Could you check a few things on this model? Use its own coordinates, in mm. A direction names the side the tool comes from. Give positions to 0.01 mm unless a question says otherwise; leave off trailing zeros. Write each question's results on one line, items separated by ' | '. Start each with the question number.
1) On a 3-axis mill with a long thin cutter (end or side, diameter ignored), from which of +Z, -Z, +X, -X, +Y, -Y can I reach the whole of each face in a straight line? I mean faces 4 (the face through (-7, 20, -320)), 5 (the face through (-7, 0, 419)). Say none if no direction works.
2) If we mould it in two halves opening along Z, with no side actions, what happens to faces 1 (the face through (-7, 20, 320)), 2 (the face through (500, 74, 7)), 3 (the face through (-7, 74, -500))? For each: +Z half, -Z half, draft (parallel to the pull), parting line (faces both ways), or undercut.
3) I'm going to push a flat-ended pin straight in: pin 1 (20 mm diameter, centred on x = 121.5, z = 324, fed in from -Y). Where does the tip first touch, or does it pass through?
4) If I drill on probe 1 along Z at (x, y) = (-83, 13); probe 2 along Y at (x, z) = (-176, 331), over which ranges is the centre line in solid material (lowest first)? Write a range as [from, to].
from build123d import *

# Parameters (mm, degrees)
ESBO_O1_W                = 1000
ESBO_O1_H                = 1000
RESSALTO_EXTRUS_O1_DEPTH = 150
ESBO_O2_W                = 40
ESBO_O2_H                = 40
CORTE_EXTRUS_O1_DEPTH    = 1001


with BuildPart() as part:
    # Esboço1 → Ressalto-extrusão1 (new body)
    with BuildSketch(Plane(origin=(0, 0, 0), x_dir=(1, 0, 0), z_dir=(0, 1, 0))):
        Rectangle(ESBO_O1_W, ESBO_O1_H)
    extrude(amount=RESSALTO_EXTRUS_O1_DEPTH)

    # Esboço2 → Corte-extrusão1 (cut, through all)
    with BuildSketch(Plane.ZY.offset(500)):
        with Locations((320, 0)):
            Rectangle(ESBO_O2_W, ESBO_O2_H)
        with Locations((-320, 0)):
            Rectangle(ESBO_O2_W, ESBO_O2_H)
    extrude(amount=-CORTE_EXTRUS_O1_DEPTH, mode=Mode.SUBTRACT)


solid = part.part
Answers:
1) face 4: +X, -X, -Y | face 5: +Z, -Z, +X, -X, -Y
2) face 1: undercut | face 2: draft | face 3: -Z half
3) pin 1: stops at y = 20
4) probe 1: z = [-500, -340], [-300, 300], [340, 500] | probe 2: y = [20, 150]
